Model file for the job. Use its own axes, mm. Face numbers are marked on the shaded views. A direction names the side the tool comes from. Coordinates: 2 decimals unless noted, no trailing zeros. Write each loop counter-clockwise with the first axis right and the second up, starting at its lowest first coordinate (ties: lowest second). Pieces come first, ordered by that corner, then holes. Notation, with made-up numbers: (-36, 89.5) -> (2, 89.5) arc R21 cw to (2, 94.5) -> close; hole circle Ø1 at (26.25, -34.75). An arc over 180 degrees is marked (long way). Write item = value, one per line. Start each with the question number.
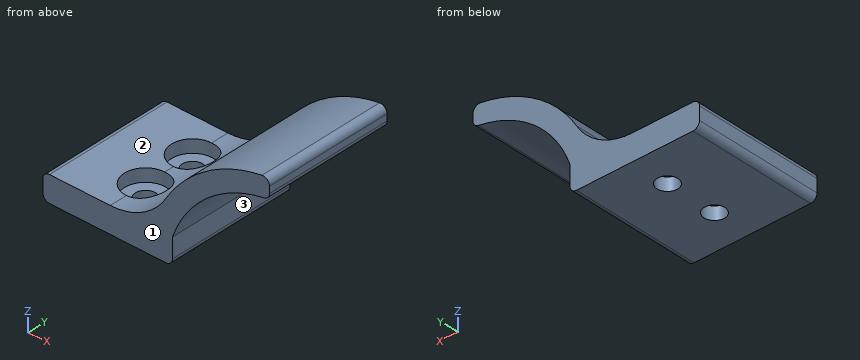
from build123d import *

# Parameters (mm, degrees)
BOSS_EXTRUDE1_DEPTH            = 20
CBORE_FOR_M3_SHCS2_D           = 3.2
CBORE_FOR_M3_SHCS2_CBORE_D     = 6.5
CBORE_FOR_M3_SHCS2_CBORE_DEPTH = 4


with BuildPart() as part:
    # Sketch1 → Boss-Extrude1 (new body)
    with BuildSketch(Plane(origin=(0, 0, 0), x_dir=(1, 0, 0), z_dir=(0, 1, 0))):
        with BuildLine():
            Line((15, -12.845583256), (15, -13.85764015))
            ThreePointArc((15, -13.85764015), (14.651920241, -14.615927695), (13.85, -14.846326147))
            ThreePointArc((13.85, -14.846326147), (5.297257748, -11.520830029), (-1.020862471, -4.865780715))
            ThreePointArc((-1.020862471, -4.865780715), (-4.669791713, -1.30108648), (-9.602225552, 0))
            Line((-9.602225552, 0), (-19, 0))
            ThreePointArc((-19, 0), (-19.707106781, 0.292893219), (-20, 1))
            Line((-20, 1), (-20, 3))
            ThreePointArc((-20, 3), (-19.707106781, 3.707106781), (-19, 4))
            Line((-19, 4), (-1, 4))
            ThreePointArc((-1, 4), (-0.292893219, 3.707106781), (0, 3))
            Line((0, 3), (0, 0))
            ThreePointArc((0, 0), (5.442271801, -7.883156387), (14.157894737, -11.858127307))
            ThreePointArc((14.157894737, -11.858127307), (14.76088591, -12.196697572), (15, -12.845583256))
        make_face()
    extrude(amount=BOSS_EXTRUDE1_DEPTH)

    # CBORE for M3 SHCS2 (through all)
    with Locations(Plane.XY.offset(2)):
        with Locations((-9.602225552, 14), (-9.602225552, 6)):
            CounterBoreHole(CBORE_FOR_M3_SHCS2_D / 2, CBORE_FOR_M3_SHCS2_CBORE_D / 2, CBORE_FOR_M3_SHCS2_CBORE_DEPTH)


solid = part.part
(1) Saw through at B-B (y = 2.25). Give the cut face in (x, z), then the cut area to 3 significant figures.
(2) Drop flat-ended pins along their axis: pin 1 Ø5 at (x, y) = (-10.5, 5) entering from +Z; pin 2 Ø1.5 at (y, z) = (8.5, 7) entering from +X; pin 3 Ø6 at (y, z) = (16, 1.5) entering from +X. Give the stop position or say it passes through.
(3) Saw through at C-C (z = 6.75). Give the cut face in (x, y), then the cut area to 3 significant figures.
(4) Saw through at A-A (y = 14). Give the cut face in (x, z).
(5) 3-axis set-ups, long thin cutter, end or side, ignore diameter. For the marked faces 1, 2 and 3: which of +Z, -Z, +X, -X, +Y, -Y reach the whole face in a straight line?
(6) Drill centre lines: line 1 along Z through (x, y) = (-16.5, 1.5); line 2 along X through (y, z) = (6, -0.15); line 3 along X through (y, z) = (7.5, 3.75). Where is each one in solid material? Low to high.
(7) Saw through at D-D (y = 11.5). Give the cut face in (x, z).
Returned:
q1.outline = (-20, -3) arc R1 ccw to (-19, -4) -> (-1, -4) arc R1 ccw to (0, -3) -> (0, 0) arc R18 cw to (14.16, 11.86) arc R1 ccw to (15, 12.85) -> (15, 13.86) arc R1 ccw to (13.85, 14.85) arc R21 ccw to (-1.02, 4.87) arc R10 cw to (-9.6, 0) -> (-19, 0) arc R1 ccw to (-20, -1) -> close
q1.area = 153 mm2
q2.pin_1 = 0
q2.pin_2 = 5.29
q2.pin_3 = 2.32
q3.outline = (0.25, 0) -> (4.21, 0) -> (4.21, 20) -> (0.25, 20) -> close
q3.area = 79.2 mm2
q4.outline = (-20, -3) arc R1 ccw to (-19, -4) -> (-11.2, -4) -> (-11.2, -2) -> (-12.85, -2) -> (-12.85, 0) -> (-19, 0) arc R1 ccw to (-20, -1) -> close; (-8, -4) -> (-1, -4) arc R1 ccw to (0, -3) -> (0, 0) arc R18 cw to (14.16, 11.86) arc R1 ccw to (15, 12.85) -> (15, 13.86) arc R1 ccw to (13.85, 14.85) arc R21 ccw to (-1.02, 4.87) arc R10 cw to (-6.35, 0.54) -> (-6.35, -2) -> (-8, -2) -> close
q5.face_1 = +Z, -Z, +X, -X, -Y
q5.face_2 = +Z, -X, +Y, -Y
q5.face_3 = -Z, +X, +Y, -Y
q6.line_1 = -4 to 0
q6.line_2 = -19.53 to -12.85, -6.35 to 0
q6.line_3 = -1.8 to 1.82
q7.outline = (-20, -3) arc R1 ccw to (-19, -4) -> (-1, -4) arc R1 ccw to (0, -3) -> (0, 0) arc R18 cw to (14.16, 11.86) arc R1 ccw to (15, 12.85) -> (15, 13.86) arc R1 ccw to (13.85, 14.85) arc R21 ccw to (-1.02, 4.87) arc R10 cw to (-7.53, 0.22) -> (-7.53, -2) -> (-11.68, -2) -> (-11.68, 0) -> (-19, 0) arc R1 ccw to (-20, -1) -> close
